from build123d import *

# Parameters (mm, degrees)
SKETCH_3_R             = 1.25
EXTRUDE_3_DEPTH        = 12
FILLET_1_R             = 3
HOLE_WIZARD_M3_1_D     = 2.5
HOLE_WIZARD_M3_1_DEPTH = 12


with BuildPart() as part:
    # 草图3 → 凸台-拉伸3 (new body)
    with BuildSketch(Plane(origin=(0, 0, 0), x_dir=(1, 0, 0), z_dir=(0, 1, 0))):
        Polygon((-68.791651246, -10.849364905), (-60.131397208, -5.849364905), (-50.131397208, -23.169872981), (-67.451905284, -33.169872981), (-72.451905284, -24.509618943), (-63.791651246, -19.509618943), align=None)
        with Locations(Location((-56.961524227, -21.339745962, 0), (0, 0, 270))):
            Circle(SKETCH_3_R, mode=Mode.SUBTRACT)
        with Locations(Location((-61.961524227, -12.679491924, 0), (0, 0, 270))):
            Circle(SKETCH_3_R, mode=Mode.SUBTRACT)
        with Locations(Location((-65.621778265, -26.339745962, 0), (0, 0, 270))):
            Circle(SKETCH_3_R, mode=Mode.SUBTRACT)
    extrude(amount=EXTRUDE_3_DEPTH)

    # 圆角1
    fillet_1_edges = [part.edges().sort_by_distance(p)[0] for p in [
        (-68.791651246, 6, 10.849364905),
        (-60.131397208, 6, 5.849364905),
        (-50.131397208, 6, 23.169872981),
        (-67.451905284, 6, 33.169872981),
        (-72.451905284, 6, 24.509618943),
        (-63.791651246, 6, 19.509618943),
    ]]
    fillet(fillet_1_edges, radius=FILLET_1_R)

    # M3 螺纹孔1
    with Locations(Plane(origin=(-61.961524227, 12, 12.679491924), x_dir=(0, 0, 1), z_dir=(0, 1, 0))):
        with Locations((0, 0), (8.660254038, 5), (13.660254038, -3.660254038)):
            Hole(HOLE_WIZARD_M3_1_D / 2, depth=HOLE_WIZARD_M3_1_DEPTH)


solid = part.part
The listing builds one solid part. Answer for the finished solid, in the listing's coordinates (mm). A direction names the side the tool comes from. Coordinates: 2 decimals unless noted, no trailing zeros. Order: outer loops, then holes, each group sorted by start corner. A loop starts at its lowest first (then second) coordinate and runs counter-clockwise, first axis right, second up. Notation, with made-up numbers: (-10.75, 29.25) -> (22.25, 29.25) arc R19 ccw to (22.25, 54.25) -> close; hole circle Ø3 at (81, -33). An arc over 180 degrees is marked (long way). Answer in a Markdown table with one row per item. Add a question column.
Item 1: Find section B-B (y = 11). Write down the section's boundary in (x, z).
Item 2: Determine the mould class of faces 1 (the face through (-64.984, 6.084, 19.156)), 2 (the face through (-61, 12, 19)), 3 (the face through (-64.568, 5.916, 27.012)) for opening direction X: +X half, -X half, draft (parallel to the pull), parting line (faces both ways), or undercut.
Item 3: Which of the six approach directions +Z, -Z, +X, -X, +Y, -Y give full straight-line access (tool end or side, diameter ignored) to faces 4 (the face through (-68.146, 5.916, 22.024)), 5 (the face through (-67, 6, 32))?
Item 4: Find the intervals of material crossed by L1, parallel to Z at x = -56.25, y = 9.25; L2, parallel to Z at x = -67, y = 8.75; L3, parallel to X at y = 5, z = 25.5, in increasing order. Write a range as from..to.
Item 5: Each of these flat-tipped pins is pushed along its axis until it touches: P1, Ø5, axis at y = 8, z = 15, coming from the -X side; P2, Ø6, axis at x = -68, y = 7, coming from the -Z side. Where does it stop, or does it pass through?
Item 6: Find section D-D (z = 28). Write down the section's boundary in (x, y), then the cut area to 3 significant figures.
Item 7: Find section A-A (x = -56). Write down the section's boundary in (y, z), then the cut area to 3 significant figures.
Item 8: Find section C-C (z = 15.25). Write down the section's boundary in (x, y), then the cut area to 3 significant figures.
Result set:
| question | item | result |
|---|---|---|
| 1 | outline | (-70.95, 27.11) arc R3 ccw to (-69.85, 23.01) -> (-66.39, 21.01) arc R3 cw to (-65.29, 16.91) -> (-67.29, 13.45) arc R3 ccw to (-66.19, 9.35) -> (-62.73, 7.35) arc R3 ccw to (-58.63, 8.45) -> (-51.63, 20.57) arc R3 ccw to (-52.73, 24.67) -> (-64.85, 31.67) arc R3 ccw to (-68.95, 30.57) -> close; hole circle Ø2.5 at (-65.62, 26.34); hole circle Ø2.5 at (-61.96, 12.68); hole circle Ø2.5 at (-56.96, 21.34) |
| 2 | face 1 | -X half |
| 2 | face 2 | draft |
| 2 | face 3 | undercut |
| 3 | face 4 | -X, +Y, -Y |
| 3 | face 5 | +Z, +Y, -Y |
| 4 | L1 | z = 12.57..20.31, 22.37..26.7 |
| 4 | L2 | z = 10.03..13.95, 21.36..32 |
| 4 | L3 | x = -71.35..-66.55, -64.7..-54.17 |
| 5 | P1 | stops at x = -67.64 |
| 5 | P2 | stops at z = 8.66 |
| 6 | outline | (-70.44, 0) -> (-58.5, 0) -> (-58.5, 12) -> (-70.44, 12) -> close |
| 6 | area | 143 mm² |
| 7 | outline | (0, 13.01) -> (12, 13.01) -> (12, 20.54) -> (0, 20.54) -> close; (0, 22.14) -> (12, 22.14) -> (12, 26.56) -> (0, 26.56) -> close |
| 7 | area | 143 mm² |
| 8 | outline | (-66.25, 0) -> (-54.7, 0) -> (-54.7, 12) -> (-66.25, 12) -> close |
| 8 | area | 139 mm² |
